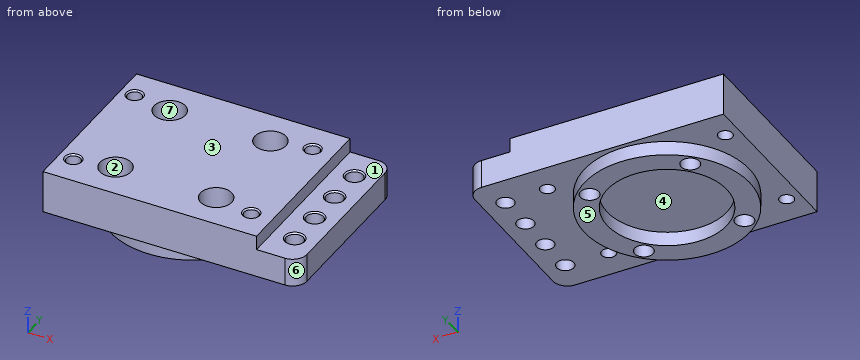
Autodesk Inventor part; units mm, degrees
ref_plane "YZ Plane" through (0, 0, 0) normal (1, 0, 0) x (0, 1, 0)
ref_plane "XZ Plane" through (0, 0, 0) normal (0, 1, 0) x (-1, 0, 0)
ref_plane "XY Plane" through (0, 0, 0) normal (0, 0, 1) x (1, 0, 0)
sketch "Sketch1" plane through (0, 0, 0) normal (0, 0, 1) x (1, 0, 0)
  circle A0 centre (510.2334, 364.1488) radius 30.5
  circle A1 centre (510.2334, 364.1488) radius 16.75
  circle A2 centre (531.1627, 350.4752) radius 3.2
  circle A3 centre (534.7013, 369.2793) radius 3.2
  circle A4 centre (505.1029, 388.6167) radius 3.2
  circle A5 centre (485.7655, 359.0183) radius 3.2
  circle A6 centre (515.3639, 339.6809) radius 3.2
  point P0 (0, 0)
extrude "Extrusion1" add sketch "Sketch1" along normal blind 10 contours A0 | A2
sketch "Sketch2" plane through (510.2334, 364.1488, 10) normal (0, 0, 1) x (1, 0, 0)
  line L0 (-40, -30.5) -> (40, -30.5)
  line L1 (40, -30.5) -> (40, 30.5)
  line L2 (40, 30.5) -> (-40, 30.5)
  line L3 (-40, 30.5) -> (-40, -30.5)
  line L4 (-40, -30.5) -> (40, 30.5) construction
  line L5 (40, -30.5) -> (-40, 30.5) construction
  circle A0 centre (0, 0) radius 30.5
  circle A1 centre (0, 0) radius 30.5
  circle A2 centre (0, 0) radius 16.75
  circle A3 centre (24.4679, 5.1305) radius 3.2
  circle A4 centre (-5.1305, 24.4679) radius 3.2
  circle A5 centre (-24.4679, -5.1305) radius 3.2
  circle A6 centre (5.1305, -24.4679) radius 3.2
  point P0 (-510.2334, -364.1488)
  point P1 (0, 0)
  dimension "d2" = 80
  dimension "d3" = 0
extrude "Extrusion2" add sketch "Sketch2" along normal blind 15
sketch "Sketch3" plane through (550.2334, 333.6488, 10) normal (1, 0, 0) x (0, 0, -1)
  line L0 (0, 0) -> (0, 61)
  line L1 (0, 61) -> (-15, 61)
  line L2 (-15, 0) -> (-15, 61)
  line L3 (0, 0) -> (-15, 0)
  line L4 (-15, 61) -> (-7.5, 61)
  line L5 (-7.5, 61) -> (-7.5, 0)
  line L6 (-7.5, 0) -> (-15, 0)
  line L7 (-15, 0) -> (-15, 61)
  line L8 (-15, 61) -> (-10, 61)
  line L9 (-10, 61) -> (-10, 0)
  line L10 (-10, 0) -> (-15, 0)
  line L11 (-15, 0) -> (-15, 61)
  point P0 (10, -333.6488)
  dimension "d34" = 5
  dimension "d35" = 15
extrude "Extrusion3" add sketch "Sketch3" along normal blind 10 contours L3 L5 L1 L0 | L3 L9 L1 L5
fillet "Fillet1" radius 5 2 edges at (560.2334, 394.6488, 15) (560.2334, 333.6488, 15)
sketch "Sketch5" plane through (510.2334, 364.1488, 25) normal (0, 0, 1) x (1, 0, 0)
  point P0 (-510.2334, -364.1488)
sketch "Sketch6" plane through (550.2334, 333.6488, 10) normal (1, 0, 0) x (0, 0, -1)
  line L0 (-10, 0) -> (-15, 0)
  line L1 (-10, 61) -> (-15, 61)
  line L2 (-15, 0) -> (-15, 61)
  line L3 (-10, 0) -> (-10, 61)
  point P0 (10, -333.6488)
extrude "Extrusion5" cut sketch "Sketch6" against normal blind 5
sketch "Sketch9" plane through (510.2334, 364.1488, 10) normal (0, 0, -1) x (-1, 0, 0)
  line L0 (-50, 30.5) -> (-35, 30.5)
  line L1 (-35, 30.5) -> (-35, -30.5)
  line L2 (-35, -30.5) -> (-50, -30.5)
  line L3 (-50, -30.5) -> (-50, 30.5)
  line L4 (-50, -25.5) -> (-50, 25.5)
  line L5 (0, 30.5) -> (-45, 30.5)
  line L6 (0, -30.5) -> (-45, -30.5)
  line L7 (-50, 30.5) -> (-42.5, 30.5)
  line L8 (-42.5, 30.5) -> (-42.5, -30.5)
  line L9 (-42.5, -30.5) -> (-50, -30.5)
  line L10 (-50, -30.5) -> (-50, 30.5)
  point P0 (510.2334, -364.1488)
  point P1 (-50, 0)
  point P2 (-42.5, -19.5)
  point P3 (-42.5, -6.5)
  point P4 (-42.5, 6.5)
  point P5 (-42.5, 19.5)
  dimension "d49" = 15
  dimension "d50" = 13
  dimension "d51" = 13
  dimension "d52" = 13
  dimension "d53" = 61
  dimension "d54" = 11
hole "Hole4" at (552.7334, 383.6488, 10) at (552.7334, 370.6488, 10) at (552.7334, 357.6488, 10) at (552.7334, 344.6488, 10) direction (0, 0, 1) diameter 6 end through all
sketch "Sketch10" plane through (510.2334, 364.1488, 25) normal (0, 0, 1) x (1, 0, 0)
  point P0 (-510.2334, -364.1488)
sketch "Sketch11" plane through (510.2334, 364.1488, 25) normal (0, 0, 1) x (1, 0, 0)
  circle A0 centre (0, 0) radius 16.75
  circle A1 centre (24.4679, 5.1305) radius 3.2
  circle A2 centre (-5.1305, 24.4679) radius 3.2
  circle A3 centre (-24.4679, -5.1305) radius 3.2
  circle A4 centre (5.1305, -24.4679) radius 3.2
  line L0 (35, -30.5) -> (35, 30.5)
  line L1 (35, 30.5) -> (-40, 30.5)
  line L2 (-40, 30.5) -> (-40, -30.5)
  line L3 (-40, -30.5) -> (35, -30.5)
  point P0 (-510.2334, -364.1488)
  point P1 (-35, 20)
  point P2 (-35, -20)
  point P3 (27.5, -20)
  point P4 (27.5, 20)
  dimension "d62" = 5
  dimension "d63" = 40
  dimension "d64" = 61
  dimension "d65" = 0
  dimension "d66" = 10.5
  dimension "d67" = 7.5
  dimension "d68" = 7.5
  dimension "d69" = 10.5
  dimension "d70" = 40
hole "Hole5" at (475.2334, 384.1488, 25) at (475.2334, 344.1488, 25) at (537.7334, 344.1488, 25) at (537.7334, 384.1488, 25) direction (0, 0, -1) diameter 5 end through all countersink diameter 6 countersink angle 90
sketch "Sketch12" plane through (510.2334, 364.1488, 25) normal (0, 0, 1) x (1, 0, 0)
  line L0 (17.6775, 17.6775) -> (-17.6775, 17.6775)
  line L1 (-17.6775, 17.6775) -> (-17.6775, -17.6775)
  line L2 (-17.6775, -17.6775) -> (17.6775, -17.6775)
  line L3 (17.6775, -17.6775) -> (17.6775, 17.6775)
  line L4 (17.6775, 17.6775) -> (-17.6775, -17.6775) construction
  line L5 (-17.6775, 17.6775) -> (17.6775, -17.6775) construction
  circle A0 centre (0, 0) radius 25
  circle A1 centre (0, 0) radius 16.75
  point P0 (-510.2334, -364.1488)
  dimension "d78" = 35.355
  dimension "d79" = 35.355
  dimension "d80" = 50
sketch "Sketch13" plane through (510.2334, 364.1488, 25) normal (0, 0, 1) x (1, 0, 0)
  circle A0 centre (27.5, 20) radius 3
  circle A1 centre (27.5, -20) radius 3
  circle A2 centre (-35, -20) radius 3
  circle A3 centre (-35, 20) radius 3
  circle A4 centre (0, 0) radius 16.75
  circle A5 centre (24.4679, 5.1305) radius 3.2
  circle A6 centre (-5.1305, 24.4679) radius 3.2
  circle A7 centre (-24.4679, -5.1305) radius 3.2
  circle A8 centre (5.1305, -24.4679) radius 3.2
  line L0 (35, -30.5) -> (35, 30.5)
  line L1 (35, 30.5) -> (-40, 30.5)
  line L2 (-40, 30.5) -> (-40, -30.5)
  line L3 (-40, -30.5) -> (35, -30.5)
  point P0 (-510.2334, -364.1488)
extrude "Extrusion6" add sketch "Sketch13" against normal up to surface (25 mm away) contours A5 | A6 | A7 | A8
sketch "Sketch14" plane through (510.2334, 364.1488, 0) normal (0, 0, -1) x (-1, 0, 0)
  circle A0 centre (0, 0) radius 30.5
  circle A1 centre (0, 0) radius 16.75
  point P0 (510.2334, -364.1488)
extrude "Extrusion7" cut sketch "Sketch14" against normal up to surface (10 mm away)
sketch "Sketch15" plane through (510.2334, 364.1488, 10) normal (0, 0, -1) x (-1, 0, 0)
  circle A0 centre (0, 0) radius 16.75
  point P0 (510.2334, -364.1488)
extrude "Extrusion8" add sketch "Sketch15" against normal up to surface (15 mm away)
sketch "Sketch16" plane through (510.2334, 364.1488, 25) normal (0, 0, 1) x (1, 0, 0)
  circle A0 centre (-3.75, 0) radius 25
  circle A1 centre (27.5, 20) radius 3
  circle A2 centre (27.5, -20) radius 3
  circle A3 centre (-35, -20) radius 3
  circle A4 centre (-35, 20) radius 3
  line L0 (35, -30.5) -> (35, 30.5)
  line L1 (35, 30.5) -> (-40, 30.5)
  line L2 (-40, 30.5) -> (-40, -30.5)
  line L3 (-40, -30.5) -> (35, -30.5)
  line L4 (-21.4277, -17.6777) -> (13.9277, -17.6777)
  line L5 (13.9277, -17.6777) -> (13.9277, 17.6777)
  line L6 (13.9277, 17.6777) -> (-21.4277, 17.6777)
  line L7 (-21.4277, 17.6777) -> (-21.4277, -17.6777)
  line L8 (-21.4277, -17.6777) -> (13.9277, 17.6777) construction
  line L9 (13.9277, -17.6777) -> (-21.4277, 17.6777) construction
  circle A5 centre (-3.75, 0) radius 29
  circle A6 centre (-3.75, 0) radius 21
  line L10 (27.5, 20) -> (-35, 20)
  line L11 (-35, 20) -> (-35, -20)
  line L12 (-35, -20) -> (27.5, -20)
  line L13 (27.5, -20) -> (27.5, 20)
  point P0 (-510.2334, -364.1488)
  dimension "d100" = 50
  dimension "d101" = 75
  dimension "d102" = 61
  dimension "d104" = 30.5
  dimension "d105" = 42
  dimension "d106" = 58
  dimension "d109" = 62.5
  dimension "d110" = 40
  dimension "d111" = 31.25
extrude "Extrusion9" add sketch "Sketch16" against normal blind 20 contours A0 L5 A6 | A0 L10 A5 L12 | L6 A6 L10 A0 | L5 A6 L6 | A0 L12 A6 L4 | L4 A6 L5 | L10 A6 A0 | A0 L10 A5 | L12 A5 A0 | A0 L12 A6 | L10 A6 L6 A0 | A0 L12 A5 L10 | A6 L7 L6 | A0 L4 A6 L12 | L4 L7 A6 | L7 A6 A0
hole "Hole7" at (488.8058, 381.8264, 25) at (488.8058, 346.4711, 25) at (524.1611, 346.4711, 25) at (524.1611, 381.8264, 25) direction (0, 0, -1) diameter 6.5 end through all counterbore diameter 11 counterbore depth 10
chamfer "Chamfer1" distance 0.5 angle 45 4 edges at (552.7334, 341.6488, 20) (552.7334, 354.6488, 20) (552.7334, 367.6488, 20) (552.7334, 380.6488, 20)
equation "\"d79\" = d78"
properties part number "UR5 gripper mount_3DPrint"
For this review, take the finished solid that the model builds, in its own axes (mm). Face numbers are marked on the shaded views. A direction names the side the tool comes from. Round coordinates to 2 decimals unless told otherwise and drop trailing zeros. Loops run counter-clockwise (first coordinate to the right, second up) from the corner with the lowest first, then second, coordinate; pieces in that order, holes last. Notation, with made-up numbers: (10.5, 20.25) - (63.5, 20.25) arc R21 cw to (63.5, 29.25) - close; hole circle Ø11 at (8, 14.5). An arc over 180 degrees is marked (long way). One line per item, written item: value. Start each with the question number.
Item 1: Clearance check with flat-ended pins moving along their axes: pin 1 Ø6.5 at (x, y) = (537.73, 384.15) entering from -Z; pin 2 Ø7.5 at (x, y) = (552.5, 373) entering from +Z; pin 3 Ø2 at (x, z) = (522.5, 8) entering from +Y; pin 4 Ø3 at (x, y) = (475.23, 344.15) entering from +Z. State where each tip first meets the part, or that it passes through.
Item 2: The part is to be moulded in two halves that separate along Y. For the marked faces 4, 5, 6 and 7, say which applies: +Y half, -Y half, draft (parallel to the pull), parting line (faces both ways), or undercut.
Item 3: Take a section at A-A (z = 18.25). State how many separate pieces and enclosed holes the cut face has, plus the area to 3 significant figures.
Item 4: Take a section at B-B (x = 490.5). Give the boundary of the cut face in (y, z), plus the area to 3 significant figures.
Item 5: For L1, parallel to X at y = 382.5, z = 21; L2, parallel to X at y = 357.5, z = 15.25; L3, parallel to Y at x = 529, z = 22, list the stretches that pass through material, from the lowest coordinate up.
Item 6: Take a section at D-D (y = 365.5). Give the boundary of the cut face in (x, z).
Item 7: For the marked faces 1, 2 and 3, list the 3-axis set-ups (+Z, -Z, +X, -X, +Y, -Y) from which the entire face can be reached by the end or side of a thin tool; tool diameter is ignored.
Answer below:
1. pin 1: stops at z = 10
1. pin 2: stops at z = 20
1. pin 3: stops at y = 388.96
1. pin 4: passes through
2. face 4: undercut
2. face 5: draft
2. face 6: -Y half
2. face 7: undercut
3. separate pieces: 1
3. enclosed holes: 12
3. area: 4,910 mm2
4. outline: (333.65, 10) - (339.95, 10) - (339.95, 5) - (343.7, 5) - (343.7, 15) - (341.24, 15) - (341.24, 25) - (333.65, 25) - close; (349.24, 5) - (350.53, 5) - (350.53, 10) - (377.77, 10) - (377.77, 5) - (379.05, 5) - (379.05, 15) - (376.59, 15) - (376.59, 25) - (351.7, 25) - (351.7, 15) - (349.24, 15) - close; (384.6, 5) - (388.35, 5) - (388.35, 10) - (394.65, 10) - (394.65, 25) - (387.06, 25) - (387.06, 15) - (384.6, 15) - close
4. area: 701 mm2
5. L1: x = 470.23 to 473.35, 477.11 to 483.35, 494.26 to 518.7, 529.62 to 535.85, 539.61 to 545.23
5. L2: x = 470.23 to 549.74, 555.73 to 560.23
5. L3: y = 333.65 to 343.86, 349.09 to 379.21, 384.44 to 394.65
6. outline: (470.23, 10) - (477.51, 10) - (477.51, 5) - (485.53, 5) - (485.53, 10) - (527.44, 10) - (527.44, 5) - (535.45, 5) - (535.45, 10) - (560.23, 10) - (560.23, 20) - (545.23, 20) - (545.23, 25) - (470.23, 25) - close
7. face 1: +Z, +X, +Y, -Y
7. face 2: +Z
7. face 3: +Z, +X, -X, +Y, -Y
